Design review of the part built by this model. Coordinates are the model's own, in mm. Round coordinates to 2 decimals unless told otherwise and drop trailing zeros. Write each loop counter-clockwise with the first axis right and the second up, starting at its lowest first coordinate (ties: lowest second). Pieces come first, ordered by that corner, then holes. Notation, with made-up numbers: (-13.5, 84.25) - (8.5, 84.25) arc R26 cw to (8.5, 123.25) - close; hole circle Ø4 at (70.25, 64.5). An arc over 180 degrees is marked (long way). Use one line per item in the form item = value.
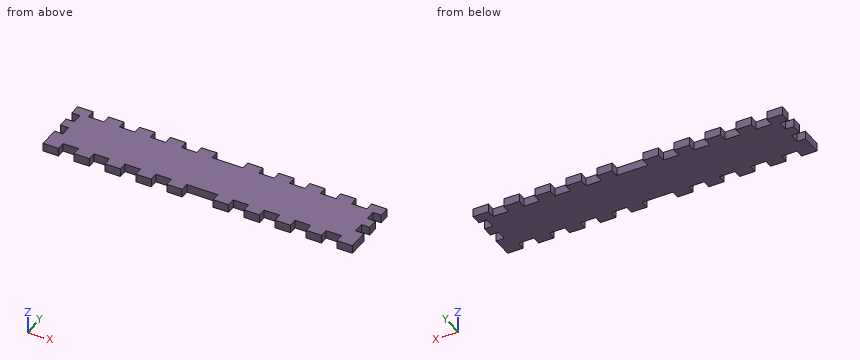
```python
from build123d import *

# Parameters (mm, degrees)
ESQUISSE1_W             = 300
ESQUISSE1_H             = 60
BOSS_EXTRU_1_DEPTH      = 8
ESQUISSE2_W             = 15
ESQUISSE2_H             = 8
ENL_V_MAT_EXTRU_1_DEPTH = 8
ESQUISSE3_W             = 8
ESQUISSE3_H             = 10
ENL_V_MAT_EXTRU_2_DEPTH = 154.179633111


with BuildPart() as part:
    # Esquisse1 → Boss.-Extru.1 (new body)
    with BuildSketch(Plane.XY):
        Rectangle(ESQUISSE1_W, ESQUISSE1_H)
    extrude(amount=BOSS_EXTRU_1_DEPTH)

    # Esquisse2 → Enlèv. mat.-Extru.1 (cut)
    with BuildSketch(Plane.XY):
        Polygon((0, -30), (15, -30), (15, -22), (0, -22), (-15, -22), (-15, -30), align=None)
        with Locations((-127.5, -26)):
            Rectangle(ESQUISSE2_W, ESQUISSE2_H)
        with Locations((-97.5, -26)):
            Rectangle(ESQUISSE2_W, ESQUISSE2_H)
        with Locations((-67.5, -26)):
            Rectangle(ESQUISSE2_W, ESQUISSE2_H)
        with Locations((-37.5, -26)):
            Rectangle(ESQUISSE2_W, ESQUISSE2_H)
        with Locations((127.5, -26)):
            Rectangle(ESQUISSE2_W, ESQUISSE2_H)
        with Locations((97.5, -26)):
            Rectangle(ESQUISSE2_W, ESQUISSE2_H)
        with Locations((67.5, -26)):
            Rectangle(ESQUISSE2_W, ESQUISSE2_H)
        with Locations((37.5, -26)):
            Rectangle(ESQUISSE2_W, ESQUISSE2_H)
    enl_v_mat_extru_1 = extrude(amount=ENL_V_MAT_EXTRU_1_DEPTH, mode=Mode.SUBTRACT)

    # Esquisse3 → Enlèv. mat.-Extru.2 (cut, through all)
    with BuildSketch(Plane.XY):
        with Locations((-146, 15)):
            Rectangle(ESQUISSE3_W, ESQUISSE3_H)
        with Locations((-146, -5)):
            Rectangle(ESQUISSE3_W, ESQUISSE3_H)
    enl_v_mat_extru_2 = extrude(amount=ENL_V_MAT_EXTRU_2_DEPTH, mode=Mode.SUBTRACT)

    # Symétrie1: Enlèv. mat.-Extru.2 across plane
    add(enl_v_mat_extru_2.mirror(Plane(origin=(0, 0, 0), x_dir=(0, 0, 1), z_dir=(1, 0, 0))), mode=Mode.SUBTRACT)

    # Symétrie2: Enlèv. mat.-Extru.1 across plane
    add(enl_v_mat_extru_1.mirror(Plane.ZX), mode=Mode.SUBTRACT)


solid = part.part
```
Q1. We need section A-A on x = 98.5. Write out the cut boundary in (y, z), then the cut area to 3 significant figures.
Calculated:
outline = (-22, 0) - (22, 0) - (22, 8) - (-22, 8) - close
area = 352 mm2
Q2. We need section B-B on y = 14.5. Write out the cut boundary in (x, z), then the cut area to 3 significant figures.
Calculated:
outline = (-142, 0) - (142, 0) - (142, 8) - (-142, 8) - close
area = 2,270 mm2
Q3. For P1, Ø4, axis at x = 68.5, z = 2.5, coming from the -Y side; P2, Ø2.5, axis at y = -6.5, z = 5, coming from the -X side; P3, Ø1.5, axis at y = 18.5, z = 4.5, coming from the +X side, all flat-tipped, find the tip position at first contact; note any pin that passes through.
Calculated:
P1 = -22
P2 = -142
P3 = 142
Q4. To check wall thickness, follow line 1 along Y through (x, z) = (-5, 7.25); line 2 along X through (y, z) = (18, 6.25). State the ranges of each line that lie inside material, in increasing order. Write a range as from..to.
Calculated:
line_1 = -22..22
line_2 = -142..142
